```python
from build123d import *

# Parameters (mm, degrees)
F1_DEPTH = 127
F3_DEPTH = 101.601
F4_W     = 79.375
F4_H     = 36.5125
F5_DEPTH = 88.9


# Not quite as in the source:
# - a feature names something its author has since deleted; it is built from what else it names


with BuildPart() as f1:
    # F0 (on Top) → F1 (new body)
    with BuildSketch(Plane.XY):
        Polygon((177.8, 0), (-177.8, 0), (-279.4, 0), (-177.8, -101.6), (177.8, -101.6), (279.4, 0), align=None)
    extrude(amount=F1_DEPTH)

    # F2 (on face) → F3 (cut, through all)
    with BuildSketch(Plane.XZ.offset(101.6)):
        with BuildLine():
            Line((19.05, 88.9), (-19.05, 88.9))
            ThreePointArc((-19.05, 88.9), (-23.5401280605, 87.0401280605), (-25.4, 82.55))
            Line((-25.4, 82.55), (-25.4, 44.45))
            ThreePointArc((-25.4, 44.45), (-23.5401280605, 39.9598719395), (-19.05, 38.1))
            Line((-19.05, 38.1), (19.05, 38.1))
            ThreePointArc((19.05, 38.1), (23.5401280605, 39.9598719395), (25.4, 44.45))
            Line((25.4, 44.45), (25.4, 82.55))
            ThreePointArc((25.4, 82.55), (23.5401280605, 87.0401280605), (19.05, 88.9))
        make_face()
    extrude(amount=-F3_DEPTH, mode=Mode.SUBTRACT)

    # F4 (on face) → F5 (cut)
    with BuildSketch(Plane.XZ.offset(101.6)):
        with Locations((-112.7125, 45.24375)):
            Rectangle(F4_W, F4_H)
        with Locations((-112.7125, 81.75625)):
            Rectangle(F4_W, F4_H)
        with Locations((112.7125, 81.75625)):
            Rectangle(F4_W, F4_H)
        with Locations((112.7125, 45.24375)):
            Rectangle(F4_W, F4_H)
    extrude(amount=-F5_DEPTH, mode=Mode.SUBTRACT)


solid = f1.part
```
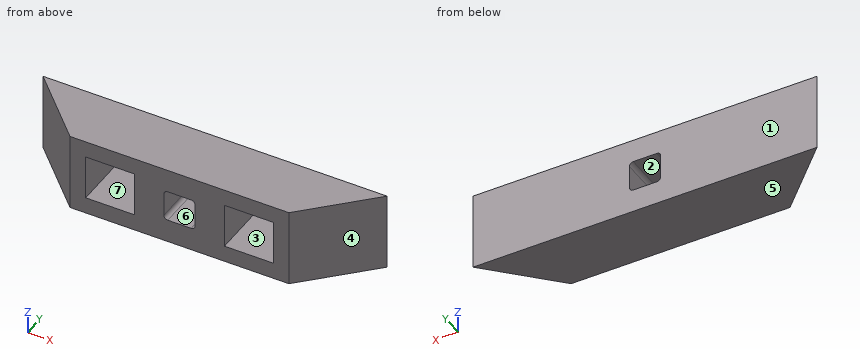
Here's how the part is built. I have some questions about the finished solid (model axes, mm). Face numbers are marked on the shaded views. A direction names the side the tool comes from. Coordinates: 2 decimals unless noted, no trailing zeros. Order: outer loops, then holes, each group sorted by start corner. A loop starts at its lowest first (then second) coordinate and runs counter-clockwise, first axis right, second up. Notation, with made-up numbers: M -6,-7 L 15,-7 A33 cw 15,31 Z; hole C -25,30 d6. An arc over 180 degrees is marked long. Answer as a JSON object with one key per item and string values. Group by question number.
(1) If we mould it in two halves opening along X, with no side actions, what happens to the marked faces 4, 5, 6 and 7? For each: released by +X, released by -X, zero draft, split by the parting line, or undercut.
(2) I need wall thicknesses on probe 1 along Z at (x, y) = (116, -79); probe 2 along X at (y, z) = (-91.5, 53) (3 decimals); probe 3 along X at (y, z) = (-52, 34) (3 decimals). Which ranges of each line are inside material? Lowest first, please.
(3) Suppose I cut it at D-D, the plane x = 0.5. Please give me the cut outline in (y, z).
(4) Suppose I cut it at B-B, the plane z = 73.5. Please give me the cut outline in (x, y) (3 decimals), then the cut area to 3 significant figures.
(5) For pin 1 (1 mm diameter, centred on y = -58, z = 33.5, fed in from +X); pin 2 (19 mm diameter, centred on y = -49, z = 60.5, fed in from -X); pin 3 (22 mm diameter, centred on x = 123, z = 53.5, fed in from -Y), each with a flat end and sliding along its axis, tell me the tip position at first contact or that it passes through.
(6) Suppose I cut it at A-A, the plane y = -45.5. State how many separate pieces and enclosed holes the cut face has, then the cut area to 3 significant figures.
(7) Suppose I cut it at C-C, the plane x = 144. Please give me the cut outline in (y, z).
(8) Which directions (+Z, -Z, +X, -X, +Y, -Y) give clear straight access to the entire face, cutting with the end or side of a thin tool? Please do the marked faces 1, 2 and 3.
Values found:
{
 "1": {"face 4": "released by +X", "face 5": "zero draft", "face 6": "undercut", "face 7": "undercut"},
 "2": {"probe 1": "z = 0 to 26.99, 100.01 to 127", "probe 2": "x = -187.9 to -152.4, -73.025 to -25.4, 25.4 to 73.025, 152.4 to 187.9", "probe 3": "x = -227.4 to -152.4, -73.025 to 73.025, 152.4 to 227.4"},
 "3": {"outline": "M -101.6,0 L 0,0 L 0,38.1 L -101.6,38.1 Z; M -101.6,88.9 L 0,88.9 L 0,127 L -101.6,127 Z"},
 "4": {"outline": "M -279.4,0 L -177.8,-101.6 L -152.4,-101.6 L -152.4,-12.7 L -73.025,-12.7 L -73.025,-101.6 L -25.4,-101.6 L -25.4,0 Z; M 25.4,-101.6 L 73.025,-101.6 L 73.025,-12.7 L 152.4,-12.7 L 152.4,-101.6 L 177.8,-101.6 L 279.4,0 L 25.4,0 Z", "area": "27,200 mm^2"},
 "5": {"pin 1": "stops at x = 221.9", "pin 2": "stops at x = -239.9", "pin 3": "stops at y = -12.7"},
 "6": {"separate pieces": "1", "enclosed holes": "3", "area": "45,300 mm^2"},
 "7": {"outline": "M -101.6,0 L 0,0 L 0,127 L -101.6,127 L -101.6,100.01 L -12.7,100.01 L -12.7,26.99 L -101.6,26.99 Z"},
 "8": {"face 1": "+Z, -Z, +X, -X, +Y", "face 2": "+Y, -Y", "face 3": "-Y"}
}
